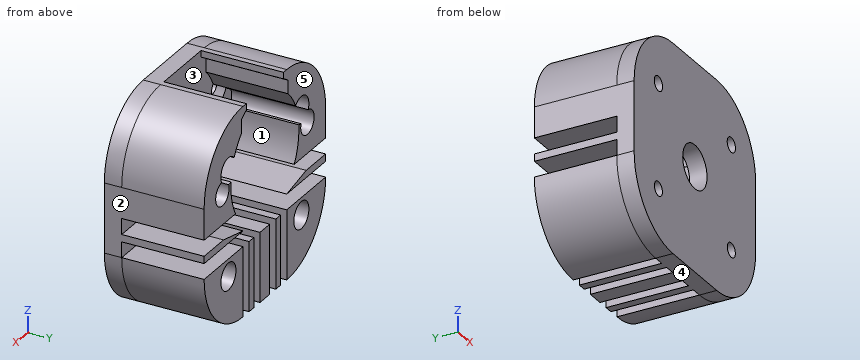
from build123d import *

# Parameters (mm, degrees)
SKETCH1_R                                    = 1.650000221024274
BOSS_EXTRUDE1_DEPTH                          = 4
BOSS_EXTRUDE2_OUTLINE_R                      = 2.75
BOSS_EXTRUDE2_OUTLINE_R_2                    = 1.650000221
BOSS_EXTRUDE2_OUTLINE_W                      = 2.000000000000001
BOSS_EXTRUDE2_OUTLINE_H                      = 16.000000209
BOSS_EXTRUDE2_OUTLINE_W_2                    = 4
BOSS_EXTRUDE2_DEPTH                          = 19
SKETCH6_R                                    = 3.1000000000000005
SKETCH6_R_2                                  = 3.0999999999999988
CUT_EXTRUDE2_DEPTH                           = 17
SKETCH7_R                                    = 3.1000000000000005
SKETCH7_R_2                                  = 3.0999999999999988
CUT_EXTRUDE3_DEPTH                           = 2
SKETCH11_R                                   = 5
CUT_EXTRUDE4_DEPTH                           = 10
CSK_FOR_M3_CROSS_RECESS_FLAT_HEAD_SC_2_COUNT = 2
CSK_FOR_M3_CROSS_RECESS_FLAT_HEAD_SC_2_PITCH = 29.999999886192118


# Read off the part's stored shape, not the designer's step: Boss-Extrude2
with BuildPart() as part:
    # Sketch1 → Boss-Extrude1 (new body)
    with BuildSketch(Plane(origin=(0, 0, 0), x_dir=(1, 0, 0), z_dir=(0, 1, 0))):
        with BuildLine():
            Line((-9.000000372528914, 24.000000208616257), (9.000000372528918, 24.000000208616257))
            ThreePointArc((9.000000372528918, 24.000000208616257), (20.31370887151379, 19.313708707601016), (25.00000037252903, 8.000000208616145))
            Line((25.00000037252903, 8.000000208616145), (25.00000037252903, -8.000000208616145))
            ThreePointArc((25.00000037252903, -8.000000208616145), (20.31370887151379, -19.313708707601016), (9.000000372528918, -24.000000208616257))
            Line((9.000000372528918, -24.000000208616257), (-9.000000372528914, -24.000000208616257))
            ThreePointArc((-9.000000372528914, -24.000000208616257), (-20.313708871513793, -19.31370870760102), (-25.00000037252903, -8.000000208616145))
            Line((-25.00000037252903, -8.000000208616145), (-25.00000037252903, 8.000000208616145))
            ThreePointArc((-25.00000037252903, 8.000000208616145), (-20.31370887151379, 19.313708707601016), (-9.000000372528914, 24.000000208616257))
        make_face()
        with Locations(Location((-14.999999943096059, 12.000001695688482, 0), (0, 0, 270))):
            Circle(SKETCH1_R, mode=Mode.SUBTRACT)
        with Locations(Location((14.999999943096059, 12.00000169568849, 0), (0, 0, 90))):
            Circle(SKETCH1_R, mode=Mode.SUBTRACT)
        with Locations(Location((14.999999943096059, -12.00000169568849, 0), (0, 0, 270))):
            Circle(SKETCH1_R, mode=Mode.SUBTRACT)
        with Locations(Location((-14.999999943096059, -12.000001695688482, 0), (0, 0, 90))):
            Circle(SKETCH1_R, mode=Mode.SUBTRACT)
    extrude(amount=BOSS_EXTRUDE1_DEPTH)

    # Boss-Extrude2 outline → Boss-Extrude2 (add)
    # profile 1 of 9: a face of its own
    with BuildSketch(Plane(origin=(0, 4, 0), x_dir=(1, 0, 0), z_dir=(0, 1, 0))):
        with BuildLine():
            ThreePointArc((-25.000000373, -8.000000209), (-20.313708872, -19.313708708), (-9.000000373, -24.000000209))
            Line((-9.000000373, -24.000000209), (-7.65, -24.000000209))
            Line((-7.65, -24.000000209), (-7.65, -22.5))
            ThreePointArc((-7.65, -22.5), (-8.646208076, -21.928947768), (-9.6, -21.289563574))
            Line((-9.6, -21.289563574), (-9.6, -18.190191362))
            ThreePointArc((-9.6, -18.190191362), (-11.86645746, -15.428807936), (-13.360259128, -12.183715576))
            ThreePointArc((-13.360259128, -12.183715576), (-16.594287762, -12.425145296), (-13.669460049, -11.024212621))
            ThreePointArc((-13.669460049, -11.024212621), (-13.83087583, -5.830466926), (-12.086943849, -0.935597096))
            Line((-12.086943849, -0.935597096), (-25.000000373, -0.935597096))
            Line((-25.000000373, -0.935597096), (-25.000000373, -8.000000209))
        make_face()
        with Locations((-17.5, -8)):
            Circle(BOSS_EXTRUDE2_OUTLINE_R, mode=Mode.SUBTRACT)
    # profile 2 of 9: a face of its own
    with BuildSketch(Plane(origin=(0, 4, 0), x_dir=(1, 0, 0), z_dir=(0, 1, 0))):
        with BuildLine():
            Line((7.65, -22.5), (7.65, -24.000000209))
            Line((7.65, -24.000000209), (9.000000373, -24.000000209))
            ThreePointArc((9.000000373, -24.000000209), (20.313708872, -19.313708708), (25.000000373, -8.000000209))
            Line((25.000000373, -8.000000209), (25.000000373, -0.935597096))
            Line((25.000000373, -0.935597096), (12.086943849, -0.935597096))
            ThreePointArc((12.086943849, -0.935597096), (13.83087583, -5.830466926), (13.669460049, -11.024212621))
            ThreePointArc((13.669460049, -11.024212621), (16.594287762, -12.425145296), (13.360259128, -12.183715576))
            ThreePointArc((13.360259128, -12.183715576), (11.86645746, -15.428807936), (9.6, -18.190191362))
            Line((9.6, -18.190191362), (9.6, -21.289563574))
            ThreePointArc((9.6, -21.289563574), (8.646208076, -21.928947768), (7.65, -22.5))
        make_face()
        with Locations((17.5, -8)):
            Circle(BOSS_EXTRUDE2_OUTLINE_R, mode=Mode.SUBTRACT)
    # profile 3 of 9: a face of its own
    with BuildSketch(Plane(origin=(0, 4, 0), x_dir=(1, 0, 0), z_dir=(0, 1, 0))):
        Polygon((-25.000000373, 4.399596768), (-25.000000373, 2.723805295), (-17, 2.723805295), (-9, 4.399596768), align=None)
    # profile 4 of 9: a face of its own
    with BuildSketch(Plane(origin=(0, 4, 0), x_dir=(1, 0, 0), z_dir=(0, 1, 0))):
        with BuildLine():
            ThreePointArc((-9.000000373, 24.000000209), (-20.313708872, 19.313708708), (-25.000000373, 8.000000209))
            Line((-25.000000373, 8.000000209), (-9, 8))
            Line((-9, 8), (-9.000000373, 24.000000209))
        make_face()
        with Locations((-14.999999943, 12.000001696)):
            Circle(BOSS_EXTRUDE2_OUTLINE_R_2, mode=Mode.SUBTRACT)
    # profile 5 of 9: a face of its own
    with BuildSketch(Plane(origin=(0, 4, 0), x_dir=(1, 0, 0), z_dir=(0, 1, 0))):
        Polygon((17, 2.723805295), (25.000000373, 2.723805295), (25.000000373, 4.399596768), (9, 4.399596768), align=None)
    # profile 6 of 9: a face of its own
    with BuildSketch(Plane(origin=(0, 4, 0), x_dir=(1, 0, 0), z_dir=(0, 1, 0))):
        with Locations((-5.5, 16.0000001045)):
            Rectangle(BOSS_EXTRUDE2_OUTLINE_W, BOSS_EXTRUDE2_OUTLINE_H)
    # profile 7 of 9: a face of its own
    with BuildSketch(Plane(origin=(0, 4, 0), x_dir=(1, 0, 0), z_dir=(0, 1, 0))):
        with BuildLine():
            Line((9, 8), (25.000000373, 8.000000209))
            ThreePointArc((25.000000373, 8.000000209), (20.313708872, 19.313708708), (9.000000373, 24.000000209))
            Line((9.000000373, 24.000000209), (9, 8))
        make_face()
        with Locations((14.999999943, 12.000001696)):
            Circle(BOSS_EXTRUDE2_OUTLINE_R_2, mode=Mode.SUBTRACT)
    # profile 8 of 9: a face of its own
    with BuildSketch(Plane(origin=(0, 4, 0), x_dir=(1, 0, 0), z_dir=(0, 1, 0))):
        with Locations((0, 16.0000001045)):
            Rectangle(BOSS_EXTRUDE2_OUTLINE_W_2, BOSS_EXTRUDE2_OUTLINE_H)
    # profile 9 of 9: a face of its own
    with BuildSketch(Plane(origin=(0, 4, 0), x_dir=(1, 0, 0), z_dir=(0, 1, 0))):
        with Locations((5.5, 16.0000001045)):
            Rectangle(BOSS_EXTRUDE2_OUTLINE_W, BOSS_EXTRUDE2_OUTLINE_H)
    extrude(amount=BOSS_EXTRUDE2_DEPTH)

    # Sketch6 → Cut-Extrude2 (cut)
    with BuildSketch(Plane(origin=(0, 23, 0), x_dir=(1, 0, 0), z_dir=(0, 1, 0))):
        with Locations((-14.999999943096059, -12.000001695688482)):
            Circle(SKETCH6_R)
        with Locations((14.999999943096062, -12.000001695688479)):
            Circle(SKETCH6_R_2)
        with Locations(Location((14.999999943096059, 12.000001695688482, 0), (0, 0, 270))):
            Circle(SKETCH6_R_2)
        with Locations(Location((-14.999999943096062, 12.000001695688479, 0), (0, 0, 90))):
            Circle(SKETCH6_R)
    extrude(amount=-CUT_EXTRUDE2_DEPTH, mode=Mode.SUBTRACT)

    # Sketch7 → Cut-Extrude3 (cut)
    with BuildSketch(Plane(origin=(0, 5.999999999999998, 0), x_dir=(1, 0, 0), z_dir=(0, 1, 0))):
        with Locations((-14.999999943096059, -12.000001695688482)):
            Circle(SKETCH7_R)
        with Locations((14.999999943096062, -12.000001695688479)):
            Circle(SKETCH7_R_2)
    extrude(amount=-CUT_EXTRUDE3_DEPTH, mode=Mode.SUBTRACT)

    # Sketch11 → Cut-Extrude4 (cut)
    with BuildSketch(Plane.XZ):
        with Locations(Location((0, 0, 0), (0, 0, 270))):
            Circle(SKETCH11_R)
    extrude(amount=-CUT_EXTRUDE4_DEPTH, mode=Mode.SUBTRACT)

    # Sketch10 → CSK for M3 Cross Recess Flat Head Screw1 (revolve, cut)
    with BuildSketch(Plane(origin=(-14.999999943096059, 4, 12.000001695688482), x_dir=(0, 0, 1), z_dir=(1, 0, 0))):
        Polygon((0, 0), (-7.6e-15, 31.021463052346846), (1.6999999999999862, 30), (1.699999999999996, 1.45), (3.15, -1.73e-15), align=None)
    csk_for_m3_cross_recess_flat_head_screw1 = revolve(axis=Axis((-14.999999943096059, 10.34999999999999, 12.000001695688482), (0, -1, 0)), mode=Mode.SUBTRACT)

    # CSK for M3 Cross Recess Flat Head Sc 2: CSK for M3 Cross Recess Flat Head Screw1 ×2
    with Locations(*[(i * CSK_FOR_M3_CROSS_RECESS_FLAT_HEAD_SC_2_PITCH, 0, 0) for i in range(1, CSK_FOR_M3_CROSS_RECESS_FLAT_HEAD_SC_2_COUNT)]):
        add(csk_for_m3_cross_recess_flat_head_screw1, mode=Mode.SUBTRACT)


solid = part.part
Geometry check sheet. Reference: the model listing, model coordinates, mm. Face numbers are marked on the shaded views. A direction names the side the tool comes from. Coordinates: 2 decimals unless noted, no trailing zeros. Order: outer loops, then holes, each group sorted by start corner. A loop starts at its lowest first (then second) coordinate and runs counter-clockwise, first axis right, second up. Notation, with made-up numbers: (22, -31.75) -> (70, -31.75) arc R22 ccw to (70, -18.75) -> close; hole circle Ø3 at (54.25, 61). An arc over 180 degrees is marked (long way). Use a Markdown table: item, result. Add a question column.
1. Cross-section at C-C (y = 1.5). Enter the section's corners in (x, z), and give its area (3 significant figures).
2. Set-up check for the marked faces 1 and 2: record each of +Z, -Z, +X, -X, +Y, -Y from which the full face is reachable in a straight line by a thin tool's end or side.
3. Go/stop test with flat-tipped pins: pin 1 Ø3 at (x, y) = (-2.5, 7) entering from +Z; pin 2 Ø6.5 at (x, y) = (-20, 12.5) entering from +Z; pin 3 Ø4.5 at (x, z) = (-15, -12) entering from +Y. Record where each tip stops, or that it passes through.
4. Cross-section at D-D (y = 19.5). Give the number of separate pieces and of enclosed holes in the cut face, and give its area (3 significant figures).
5. Material ranges on L1, parallel to Z at x = -10, y = 10.25; L2, parallel to Z at x = -17.5, y = 17; L3, parallel to Z at x = 15, y = 1.05, recorded low to high.
6. Cross-section at B-B (z = 0). Enter the section's corners in (x, y).
7. Mould release check, pull along Z, two halves, no side actions. Record for the marked faces 3, 4 and 5: pulls with the +Z half, pulls with the -Z half, needs draft (parallel to the pull), parting line crosses it, or undercut.
8. Cross-section at A-A (x = 0). Enter the section's corners in (y, z), and give its area (3 significant figures).
Filled sheet:
| question | item | result |
|---|---|---|
| 1 | outline | (-25, -8) arc R16 ccw to (-9, -24) -> (9, -24) arc R16 ccw to (25, -8) -> (25, 8) arc R16 ccw to (9, 24) -> (-9, 24) arc R16 ccw to (-25, 8) -> close; hole circle Ø3.4 at (-15, 12); hole circle Ø3.3 at (-15, -12); hole circle Ø10 at (0, 0); hole circle Ø3.4 at (15, 12); hole circle Ø3.3 at (15, -12) |
| 1 | area | 2,070 mm2 |
| 2 | face 1 | +Y |
| 2 | face 2 | +Z, -Z, +X, +Y, -Y |
| 3 | pin 1 | z = -8 |
| 3 | pin 2 | z = 22 |
| 3 | pin 3 | y = 6 |
| 4 | separate pieces | 9 |
| 4 | enclosed holes | 2 |
| 4 | area | 912 mm2 |
| 5 | L1 | -23.97 to -8, -4.4 to -4.19, 17.8 to 23.97 |
| 5 | L2 | -21.56 to -13.83, -10.17 to -8, -4.4 to -2.72, 0.94 to 5.25, 13.83 to 21.56 |
| 5 | L3 | -22.83 to -13.65, -10.35 to 10.3, 13.7 to 22.83 |
| 6 | outline | (-25, 0) -> (-5, 0) -> (-5, 4) -> (-25, 4) -> close; (5, 0) -> (25, 0) -> (25, 4) -> (5, 4) -> close |
| 7 | face 3 | undercut |
| 7 | face 4 | pulls with the -Z half |
| 7 | face 5 | needs draft |
| 8 | outline | (0, -24) -> (23, -24) -> (23, -8) -> (4, -8) -> (4, -5) -> (0, -5) -> close; (0, 5) -> (4, 5) -> (4, 24) -> (0, 24) -> close |
| 8 | area | 456 mm2 |
